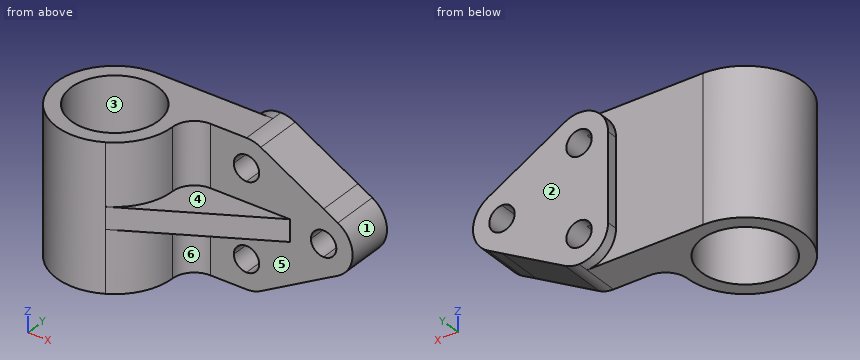
from build123d import *

# Parameters (mm, degrees)
F0_R     = 19.05
F1_DEPTH = 31.75
F2_DEPTH = 4.7625
F4_R     = 5.5626
F5_DEPTH = 20.6502
F6_DEPTH = 55.5762


with BuildPart() as f1:
    # F0 (on Top) → F1 (new body, symmetric)
    with BuildSketch(Plane.XY):
        with BuildLine():
            ThreePointArc((12.269125, -22.240247), (21.872309, -12.913641), (25.4, 0))
            ThreePointArc((25.4, 0), (28.189808, 6.735192), (34.925, 9.525))
            Line((34.925, 9.525), (69.85, 9.525))
            Line((69.85, 9.525), (84.582, 9.525))
            Line((84.582, 9.525), (84.582, 30.1752))
            Line((84.582, 30.1752), (50.8, 30.1752))
            Line((50.8, 30.1752), (50.8, 25.4))
            Line((50.8, 25.4), (0, 25.4))
            ThreePointArc((0, 25.4), (-24.597381, -6.334735), (12.269125, -22.240247))
        make_face()
        Circle(F0_R, mode=Mode.SUBTRACT)
    extrude(amount=F1_DEPTH, both=True)

    # F0 (on Top) → F2 (join, symmetric)
    with BuildSketch(Plane.XY):
        with BuildLine():
            ThreePointArc((34.925, 9.525), (28.189808, 6.735192), (25.4, 0))
            ThreePointArc((25.4, 0), (21.872309, -12.913641), (12.269125, -22.240247))
            Line((12.269125, -22.240247), (69.85, 9.525))
            Line((69.85, 9.525), (34.925, 9.525))
        make_face()
    extrude(amount=F2_DEPTH, both=True)

    # F4 (on face) → F5 (join)
    with BuildSketch(Plane(origin=(0, 30.1752, 0), x_dir=(-1, 0, 0), z_dir=(0, 1, 0))):
        with BuildLine():
            Line((-38.1, -19.05), (-38.1, 19.05))
            ThreePointArc((-38.1, 19.05), (-44.394325, 30.01619), (-57.038161, 30.112339))
            Line((-57.038161, 30.112339), (-90.820161, 11.062339))
            ThreePointArc((-90.820161, 11.062339), (-97.282, 0), (-90.820161, -11.062339))
            Line((-90.820161, -11.062339), (-57.038161, -30.112339))
            ThreePointArc((-57.038161, -30.112339), (-44.394325, -30.01619), (-38.1, -19.05))
        make_face()
        with Locations((-50.8, -19.05)):
            Circle(F4_R, mode=Mode.SUBTRACT)
        with Locations((-84.582, 0)):
            Circle(F4_R, mode=Mode.SUBTRACT)
        with Locations((-50.8, 19.05)):
            Circle(F4_R, mode=Mode.SUBTRACT)
    extrude(amount=-F5_DEPTH)

    # F4 (on face) → F6 (cut, through all)
    with BuildSketch(Plane(origin=(0, 30.1752, 0), x_dir=(-1, 0, 0), z_dir=(0, 1, 0))):
        with BuildLine():
            ThreePointArc((-45.2374, -19.05), (-46.866648, -15.116648), (-50.8, -13.4874))
            Line((-50.8, -13.4874), (-50.8, -24.6126))
            ThreePointArc((-50.8, -24.6126), (-46.866648, -22.983352), (-45.2374, -19.05))
        make_face()
        with BuildLine():
            Line((-50.8, 13.4874), (-50.8, 24.6126))
            ThreePointArc((-50.8, 24.6126), (-56.3626, 19.05), (-50.8, 13.4874))
        make_face()
        with BuildLine():
            ThreePointArc((-79.0194, 0), (-80.648648, 3.933352), (-84.582, 5.5626))
            Line((-84.582, 5.5626), (-84.582, -5.5626))
            ThreePointArc((-84.582, -5.5626), (-80.648648, -3.933352), (-79.0194, 0))
        make_face()
        with BuildLine():
            ThreePointArc((-50.8, 13.4874), (-46.866648, 15.116648), (-45.2374, 19.05))
            ThreePointArc((-45.2374, 19.05), (-46.866648, 22.983352), (-50.8, 24.6126))
            Line((-50.8, 24.6126), (-50.8, 13.4874))
        make_face()
        with BuildLine():
            Line((-50.8, -24.6126), (-50.8, -13.4874))
            ThreePointArc((-50.8, -13.4874), (-56.3626, -19.05), (-50.8, -24.6126))
        make_face()
        with BuildLine():
            ThreePointArc((-57.038161, 30.112339), (-54.024771, 31.333764), (-50.8, 31.75))
            Line((-50.8, 31.75), (-84.582, 31.75))
            Line((-84.582, 31.75), (-84.582, 14.580099))
            Line((-84.582, 14.580099), (-57.038161, 30.112339))
        make_face()
        with BuildLine():
            Line((-84.582, -31.75), (-50.8, -31.75))
            ThreePointArc((-50.8, -31.75), (-54.024771, -31.333764), (-57.038161, -30.112339))
            Line((-57.038161, -30.112339), (-84.582, -14.580099))
            Line((-84.582, -14.580099), (-84.582, -31.75))
        make_face()
    extrude(amount=-F6_DEPTH, mode=Mode.SUBTRACT)


solid = f1.part
The model under review builds one solid part; all positions refer to its coordinate system, in mm. Face numbers are marked on the shaded views. A direction names the side the tool comes from. Coordinates: 2 decimals unless noted, no trailing zeros. Write each loop counter-clockwise with the first axis right and the second up, starting at its lowest first coordinate (ties: lowest second). Pieces come first, ordered by that corner, then holes. Notation, with made-up numbers: (88, 27) - (117, 27) arc R10 cw to (117, 42) - close; hole circle Ø8 at (-5, 76.25). An arc over 180 degrees is marked (long way). Answer as a JSON object with one key per item and string values. Group by question number.
1. Add section C-C (x = 2.5). Give the boundary of the cut face in (y, z).
2. Add section D-D (y = 22.5). Give the boundary of the cut face in (x, z), plus the area to 3 significant figures.
3. To check wall thickness, follow probe 1 along Z at (x, y) = (50.8, 23.25); probe 2 along X at (y, z) = (22.75, 19.05); probe 3 along Y at (x, z) = (0, 4.5). State the ranges of each line that lie inside material, in increasing order.
4. Mouldability with a two-part tool opening along X and no side actions: class the marked faces 1, 2 and 3 as pulls with the +X half, pulls with the -X half, needs draft (parallel to the pull), parting line crosses it, or undercut.
5. Add section B-B (z = 23). Give the boundary of the cut face in (x, y) (3 decimals), plus the area to 3 significant figures.
6. Machinability: for the marked faces 4, 5 and 6, which of the approach directions +Z, -Z, +X, -X, +Y, -Y give a long, thin tool a straight path to every point of the face, cutting with its end or side? Answer none if there is none.
7. Clearance check with flat-ended pins moving along their axes: pin 1 Ø4 at (y, z) = (28, -4) entering from -X; pin 2 Ø14.5 at (x, z) = (50.8, 19.05) entering from +Y; pin 3 Ø1 at (y, z) = (-6.5, -17.5) entering from +X; pin 4 Ø8 at (x, z) = (-0.5, -20.5) entering from +Y. State where each tip first meets the part, or that it passes through.
8. Add section A-A (y = 8). Give the boundary of the cut face in (x, z), plus the area to 3 significant figures.
Findings:
{
 "1": {"outline": "(-25.28, -31.75) - (-18.89, -31.75) - (-18.89, 31.75) - (-25.28, 31.75) - close; (18.89, -31.75) - (25.4, -31.75) - (25.4, 31.75) - (18.89, 31.75) - close"},
 "2": {"outline": "(-11.79, -31.75) - (50.8, -31.75) arc R12.7 ccw to (57.04, -30.11) - (90.82, -11.06) arc R12.7 ccw to (90.82, 11.06) - (57.04, 30.11) arc R12.7 ccw to (50.8, 31.75) - (-11.79, 31.75) - close; hole circle Ø11.13 at (50.8, -19.05); hole (45.24, 19.05) arc R5.56 ccw (long way) to (50.8, 24.61) arc R5.56 ccw to start; hole (79.02, 0) arc R5.56 ccw (long way) to (84.58, 5.56) arc R5.56 ccw to start", "area": "5,560 mm²"},
 "3": {"probe 1": "-31.75 to -24.61, -13.49 to 13.49, 24.61 to 31.75", "probe 2": "-11.3 to 45.24, 56.36 to 76.66", "probe 3": "-25.4 to -19.05, 19.05 to 25.4"},
 "4": {"face 1": "pulls with the +X half", "face 2": "needs draft", "face 3": "undercut"},
 "5": {"outline": "(0, 25.4) arc R25.4 ccw (long way) to (12.269, -22.24) arc R25.4 ccw to (25.4, 0) arc R9.525 cw to (34.925, 9.525) - (46.883, 9.525) - (46.883, 30.175) - (38.73, 30.175) - (38.73, 25.4) - close; (54.717, 9.525) - (69.651, 9.525) - (69.651, 30.175) - (54.717, 30.175) - close; hole circle Ø38.1 at (0, 0)", "area": "1,730 mm²"},
 "6": {"face 4": "+Z, +X, -Y", "face 5": "+X, -Y", "face 6": "-Z, +X, -Y"},
 "7": {"pin 1": "x = 38.1", "pin 2": "y = 30.18", "pin 3": "x = 24.68", "pin 4": "y = 25.4"},
 "8": {"outline": "(-24.11, -31.75) - (-17.29, -31.75) - (-17.29, 31.75) - (-24.11, 31.75) - close; (17.29, -31.75) - (29.76, -31.75) - (29.76, -4.76) - (67.09, -4.76) - (67.09, 4.76) - (29.76, 4.76) - (29.76, 31.75) - (17.29, 31.75) - close", "area": "1,580 mm²"}
}
